Here's how the part is built. I have some questions about the finished solid (model axes, mm). Face numbers are marked on the shaded views. A direction names the side the tool comes from. Coordinates: 2 decimals unless noted, no trailing zeros. Write each loop counter-clockwise with the first axis right and the second up, starting at its lowest first coordinate (ties: lowest second). Pieces come first, ordered by that corner, then holes. Notation, with made-up numbers: M 84.5,37 L 115.5,37 A24 ccw 115.5,76 Z; hole C -32.75,76 d4. An arc over 180 degrees is marked long. Use a Markdown table: item, result.
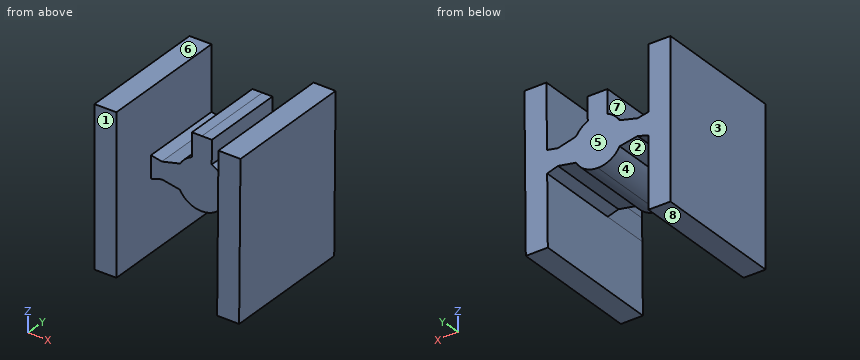
```python
from build123d import *

# Parameters (mm, degrees)
BOSS_EXTRUDE1_DEPTH     = 33
CUT_EXTRUDE1_DEPTH      = 83.954293528
CUT_EXTRUDE1_DEPTH_BACK = 12
SKETCH3_W               = 9.481209811
SKETCH3_H               = 17.021727652
CUT_EXTRUDE2_DEPTH      = 22


with BuildPart() as part:
    # Sketch1 → Boss-Extrude1 (new body)
    with BuildSketch(Plane(origin=(0, 0, 0), x_dir=(1, 0, 0), z_dir=(0, 1, 0))):
        with BuildLine():
            Line((27.99701897, 26.104397373), (30.497019389, 26.104397373))
            Line((30.497019389, 26.104397373), (32.996926828, 26.125958592))
            Line((32.996926828, 26.125958592), (32.946330796, 31.992296402))
            ThreePointArc((32.946330796, 31.992296402), (34.614300355, 33.056919945), (35.86386473, 34.591238885))
            Line((35.86386473, 34.591238885), (40.431539769, 35.753760832))
            Line((40.431539769, 35.753760832), (43.136211097, 35.223788843))
            Line((43.136211097, 35.223788843), (43.274382132, 19.203600277))
            Line((43.274382132, 19.203600277), (48.774177579, 19.251034952))
            Line((48.774177579, 19.251034952), (48.43630867, 58.425118026))
            Line((48.43630867, 58.425118026), (42.936513223, 58.377683351))
            Line((42.936513223, 58.377683351), (43.088196039, 40.790876563))
            Line((43.088196039, 40.790876563), (40.395268448, 39.959225491))
            Line((40.395268448, 39.959225491), (35.888631414, 40.775372904))
            ThreePointArc((35.888631414, 40.775372904), (33.583892359, 43.097075019), (30.420151943, 43.929462788))
            ThreePointArc((30.420151943, 43.929462788), (27.263708108, 43.06982034), (24.979078258, 40.728327384))
            Line((24.979078258, 40.728327384), (20.479647685, 39.873342894))
            Line((20.479647685, 39.873342894), (17.779647685, 40.681737919))
            Line((17.779647685, 40.681737919), (17.779647685, 58.269198812))
            Line((17.779647685, 58.269198812), (12.279647685, 58.269198812))
            Line((12.279647685, 58.269198812), (12.279647685, 19.093658738))
            Line((12.279647685, 19.093658738), (17.779647685, 19.093658738))
            Line((17.779647685, 19.093658738), (17.779647685, 35.114443143))
            Line((17.779647685, 35.114443143), (20.479647685, 35.667721822))
            Line((20.479647685, 35.667721822), (25.057179, 34.544636961))
            ThreePointArc((25.057179, 34.544636961), (26.319929615, 33.021151936), (27.99701897, 31.970953369))
            Line((27.99701897, 31.970953369), (27.99701897, 26.104397373))
        make_face()
    extrude(amount=BOSS_EXTRUDE1_DEPTH)

    # Sketch2 → Cut-Extrude1 (cut, two sides: drawn at the far end of the back side and taken through both)
    with BuildSketch(Plane.XZ.offset(-CUT_EXTRUDE1_DEPTH_BACK)):
        with BuildLine():
            Line((20.479647685, -35.667721822), (17.779647685, -35.114443143))
            Line((17.779647685, -35.114443143), (17.779647685, -40.681737919))
            Line((17.779647685, -40.681737919), (20.479647685, -39.873342894))
            Line((20.479647685, -39.873342894), (24.979078258, -40.728327384))
            ThreePointArc((24.979078258, -40.728327384), (27.263708108, -43.06982034), (30.420151943, -43.929462788))
            ThreePointArc((30.420151943, -43.929462788), (33.576595778, -43.084424394), (35.888631414, -40.775372904))
            Line((35.888631414, -40.775372904), (40.395268448, -39.959225491))
            Line((40.395268448, -39.959225491), (43.088196039, -40.790876563))
            Line((43.088196039, -40.790876563), (43.136211097, -35.223788843))
            Line((43.136211097, -35.223788843), (40.431539769, -35.753760832))
            Line((40.431539769, -35.753760832), (35.86386473, -34.591238885))
            ThreePointArc((35.86386473, -34.591238885), (34.614300355, -33.056919945), (32.946330796, -31.992296402))
            Line((32.946330796, -31.992296402), (32.996926828, -26.125958592))
            Line((32.996926828, -26.125958592), (27.99701897, -26.104397373))
            Line((27.99701897, -26.104397373), (27.99701897, -31.970953369))
            ThreePointArc((27.99701897, -31.970953369), (26.319929615, -33.021151936), (25.057179, -34.544636961))
            Line((25.057179, -34.544636961), (20.479647685, -35.667721822))
        make_face()
    extrude(amount=CUT_EXTRUDE1_DEPTH + CUT_EXTRUDE1_DEPTH_BACK, mode=Mode.SUBTRACT)

    # Sketch3 → Cut-Extrude2 (cut)
    with BuildSketch(Plane.XY.offset(-26.104397373)):
        with Locations((32.737623876, 3.489136174)):
            Rectangle(SKETCH3_W, SKETCH3_H)
    extrude(amount=-CUT_EXTRUDE2_DEPTH, mode=Mode.SUBTRACT)


solid = part.part
```
1. Suppose I cut it at B-B on z = -29.5. Write out the boundary of the cut face in (x, y), and give its area (3 significant figures).
Answers follow:
| item | result |
|---|---|
| outline | M 12.28,0 L 17.78,0 L 17.78,33 L 12.28,33 Z; M 28,12 L 32.97,12 L 32.97,33 L 28,33 Z; M 43.19,0 L 48.69,0 L 48.69,33 L 43.19,33 Z |
| area | 467 mm2 |
2. Suppose I cut it at A-A on y = 9. Write out the boundary of the cut face in (x, z).
Answers follow:
| item | result |
|---|---|
| outline | M 12.28,-58.27 L 17.78,-58.27 L 17.78,-19.09 L 12.28,-19.09 Z; M 42.94,-58.38 L 48.44,-58.43 L 48.77,-19.25 L 43.27,-19.2 Z |
3. Suppose I cut it at C-C on y = 18. Write out the boundary of the cut face in (x, z), and give its area (3 significant figures).
Answers follow:
| item | result |
|---|---|
| outline | M 12.28,-58.27 L 17.78,-58.27 L 17.78,-40.68 L 20.48,-39.87 L 24.98,-40.73 A6.22 ccw 30.42,-43.93 A6.22 ccw 35.89,-40.78 L 40.4,-39.96 L 43.09,-40.79 L 42.94,-58.38 L 48.44,-58.43 L 48.77,-19.25 L 43.27,-19.2 L 43.14,-35.22 L 40.43,-35.75 L 35.86,-34.59 A6.22 ccw 32.95,-31.99 L 33,-26.13 L 30.5,-26.1 L 28,-26.1 L 28,-31.97 A6.22 ccw 25.06,-34.54 L 20.48,-35.67 L 17.78,-35.11 L 17.78,-19.09 L 12.28,-19.09 Z |
| area | 648 mm2 |
4. Which directions (+Z, -Z, +X, -X, +Y, -Y) give clear straight access to the entire face, cutting with the end or side of a thin tool? Please do the marked faces 4, 5, 6, 7 and 8.
Answers follow:
| item | result |
|---|---|
| face 4 | -Z, +Y, -Y |
| face 5 | +Z, -Z, +X, -X, +Y |
| face 6 | +Z, +X, -X, +Y, -Y |
| face 7 | +Z, +Y, -Y |
| face 8 | -Z, -X, +Y, -Y |
5. We'd pull the mould along X, two halves only. Please class the marked faces 1, 2 and 3: +X half, -X half, draft (parallel to the pull), parting line (faces both ways), or undercut.
Answers follow:
| item | result |
|---|---|
| face 1 | draft |
| face 2 | undercut |
| face 3 | -X half |
6. Will these pins go through, and if not, where does the flat tip stop? pin 1 Ø9 at (x, z) = (30, -32) entering from -Y; pin 2 Ø3 at (x, y) = (27, 15.5) entering from +Z; pin 3 Ø3 at (x, y) = (16, 23.5) entering from -Z.
Answers follow:
| item | result |
|---|---|
| pin 1 | stops at y = 12 |
| pin 2 | stops at z = -26.1 |
| pin 3 | stops at z = -58.27 |
7. Suppose I cut it at D-D on z = -24. Write out the boundary of the cut face in (x, y).
Answers follow:
| item | result |
|---|---|
| outline | M 12.28,0 L 17.78,0 L 17.78,33 L 12.28,33 Z; M 43.23,0 L 48.73,0 L 48.73,33 L 43.23,33 Z |
8. I need wall thicknesses on probe 1 along X at (y, z) = (26.5, -28); probe 2 along X at (y, z) = (29, -42.5); probe 3 along X at (y, z) = (4, -50). Which ranges of each line are inside material? Lowest first, please.
Answers follow:
| item | result |
|---|---|
| probe 1 | x = 12.28 to 17.78, 28 to 32.98, 43.2 to 48.7 |
| probe 2 | x = 12.28 to 17.78, 26.45 to 34.44, 43.07 to 48.57 |
| probe 3 | x = 12.28 to 17.78, 43.01 to 48.51 |
